Design review of the part built by this model. Coordinates are the model's own, in mm. A direction names the side the tool comes from. Coordinates: 2 decimals unless noted, no trailing zeros. Loops run counter-clockwise (first coordinate to the right, second up) from the corner with the lowest first, then second, coordinate; pieces in that order, holes last. Notation, with made-up numbers: (67.25, 86.5) -> (125.25, 86.5) arc R12 ccw to (125.25, 101.5) -> close; hole circle Ø7 at (56, 14). An arc over 180 degrees is marked (long way). Use CSV: the item, a comma, the result in double quotes.
```python
from build123d import *

# Parameters (mm, degrees)
CIRKEL_R                   = 17
CILINDER_DEPTH             = 20
CIRKEL_GAT_R               = 5.1
OPENING_DEPTH              = 10
GATEN_PATROON_COUNT        = 3
CIRKEL1_R                  = 13.5
OPENING_OPZET_DEPTH        = 3
CIRKEL2_R                  = 1.9
GAT_VERLOOPSTUK_DEPTH      = 8
CIRKEL3_R                  = 2.9
GAT_VERLOOPSTUK_RAND_DEPTH = 2


with BuildPart() as part:
    # cirkel → cilinder (new body)
    with BuildSketch(Plane(origin=(0, 0, 0), x_dir=(1, 0, 0), z_dir=(0, 1, 0))):
        with Locations(Location((0, 0, 0), (0, 0, 270))):
            Circle(CIRKEL_R)
    extrude(amount=CILINDER_DEPTH)

    # cirkel_gat → opening (cut)
    with BuildSketch(Plane.XY.offset(17)):
        with Locations((0, 10)):
            Circle(CIRKEL_GAT_R)
    opening = extrude(amount=-OPENING_DEPTH, mode=Mode.SUBTRACT)

    # gaten_patroon: opening ×3 about axis
    gaten_patroon_axis = Axis((0, 0, 0), (0, 1, 0))
    for i in range(1, GATEN_PATROON_COUNT):
        add(opening.rotate(gaten_patroon_axis, i * 360 / GATEN_PATROON_COUNT), mode=Mode.SUBTRACT)

    # cirkel1 → opening_opzet (cut)
    with BuildSketch(Plane(origin=(0, 0, 0), x_dir=(-1, 0, 0), z_dir=(0, -1, 0))):
        with Locations(Location((0, 0, 0), (0, 0, 90))):
            Circle(CIRKEL1_R)
    extrude(amount=-OPENING_OPZET_DEPTH, mode=Mode.SUBTRACT)

    # cirkel2 → gat_verloopstuk (cut)
    with BuildSketch(Plane(origin=(0, 3, 0), x_dir=(-1, 0, 0), z_dir=(0, -1, 0))):
        with Locations(Location((0, 0, 0), (0, 0, 90))):
            Circle(CIRKEL2_R)
    extrude(amount=-GAT_VERLOOPSTUK_DEPTH, mode=Mode.SUBTRACT)

    # cirkel3 → gat_verloopstuk_rand (cut)
    with BuildSketch(Plane.XZ.offset(-3)):
        with Locations(Location((0, 0, 0), (0, 0, 270))):
            Circle(CIRKEL3_R)
    extrude(amount=-GAT_VERLOOPSTUK_RAND_DEPTH, mode=Mode.SUBTRACT)


solid = part.part
```
Item 1: To check wall thickness, follow line 1 along X through (y, z) = (4.35, 0); line 2 along X through (y, z) = (1.95, 0); line 3 along Y through (x, z) = (-11, -2). State the ranges of each line that lie inside material, in increasing order.
Checked values:
line 1,"-17 to -2.9, 2.9 to 17"
line 2,"-17 to -13.5, 13.5 to 17"
line 3,"3 to 6.56, 13.44 to 20"
Item 2: Machinability: for faces 4 (the face through (-1, 15, 12)), 5 (the face through (-0.728, 7.958, -1.755)), 6 (the face through (-6.026, 10.071, -3.562)), which of the approach directions +Z, -Z, +X, -X, +Y, -Y give a long, thin tool a straight path to every point of the face, cutting with its end or side? Answer none if there is none.
Checked values:
face 4,"+Z"
face 5,"-Y"
face 6,"none"
Item 3: Add section A-A (x = 0). Give the boundary of the cut face in (y, z), then the cut area to 3 significant figures.
Checked values:
outline,"(0, -17) -> (20, -17) -> (20, 17) -> (15.1, 17) -> (15.1, 7) -> (4.9, 7) -> (4.9, 17) -> (0, 17) -> (0, 13.5) -> (3, 13.5) -> (3, 2.9) -> (5, 2.9) -> (5, 1.9) -> (11, 1.9) -> (11, -1.9) -> (5, -1.9) -> (5, -2.9) -> (3, -2.9) -> (3, -13.5) -> (0, -13.5) -> close"
area,"463 mm^2"
Item 4: Add section D-D (z = -1). State how many separate pieces and enclosed holes the cut face has, then the cut area to 3 significant figures.
Checked values:
separate pieces,"1"
enclosed holes,"2"
area,"515 mm^2"
Item 5: Draft analysis for pull direction X (two halves, no side actions). For faces 1 (the face through (0, 11, 0)), 2 (the face through (0, 20, 0)), 3 (the face through (16.855, 9.86, -2.213)), state which applies: pulls with the +X half, pulls with the -X half, needs draft (parallel to the pull), parting line crosses it, or undercut.
Checked values:
face 1,"undercut"
face 2,"needs draft"
face 3,"parting line crosses it"
Item 6: Clearance check with flat-ended pins moving along their axes: pin 1 (2 mm diameter, centred on x = 9.5, y = 14.5, fed in from +Z); pin 2 (6 mm diameter, centred on y = 15, z = 5.5, fed in from +X); pin 3 (2 mm diameter, centred on x = -7, y = 3, fed in from +Z). State where each tip first meets the part, or that it passes through.
Checked values:
pin 1,"z = 14.72"
pin 2,"x = 16.82"
pin 3,"z = 15.91"
Item 7: Add section C-C (y = 14.5). Give the boundary of the cut face in (x, z).
Checked values:
outline,"(-15.77, -6.34) -> (-7.26, -1.42) -> (-4.86, -5.58) -> (-13.37, -10.49) arc R17 ccw to (13.37, -10.49) -> (4.86, -5.58) -> (7.26, -1.42) -> (15.77, -6.34) arc R17 ccw to (2.4, 16.83) -> (2.4, 7) -> (-2.4, 7) -> (-2.4, 16.83) arc R17 ccw to start"
Item 8: Add section B-B (y = 10). Give the boundary of the cut face in (x, z), then the cut area to 3 significant figures.
Checked values:
outline,"(-16.59, -3.69) -> (-8.61, 0.92) -> (-3.51, -7.92) -> (-11.49, -12.53) arc R17 ccw to (11.49, -12.53) -> (3.51, -7.92) -> (8.61, 0.92) -> (16.59, -3.69) arc R17 ccw to (5.1, 16.22) -> (5.1, 7) -> (-5.1, 7) -> (-5.1, 16.22) arc R17 ccw to start; hole circle Ø3.8 at (0, 0)"
area,"598 mm^2"
